```python
from build123d import *

# Parameters (mm, degrees)
SKETCH1_W           = 76.2
SKETCH1_H           = 101.6
SKETCH1_R           = 2.25
BOSS_EXTRUDE1_DEPTH = 3.175


with BuildPart() as part:
    # Sketch1 → Boss-Extrude1 (new body)
    with BuildSketch(Plane(origin=(0, 0, 0), x_dir=(1, 0, 0), z_dir=(0, 1, 0))):
        Rectangle(SKETCH1_W, SKETCH1_H)
        with Locations((-19.05, -41.275)):
            Circle(SKETCH1_R, mode=Mode.SUBTRACT)
        with Locations((19.05, -41.275)):
            Circle(SKETCH1_R, mode=Mode.SUBTRACT)
        with Locations((28.575, -35.56)):
            Circle(SKETCH1_R, mode=Mode.SUBTRACT)
        with Locations((-28.575, -35.56)):
            Circle(SKETCH1_R, mode=Mode.SUBTRACT)
        with Locations((28.575, 35.56)):
            Circle(SKETCH1_R, mode=Mode.SUBTRACT)
        with Locations((19.05, 41.275)):
            Circle(SKETCH1_R, mode=Mode.SUBTRACT)
        with Locations((-28.575, 35.56)):
            Circle(SKETCH1_R, mode=Mode.SUBTRACT)
        with Locations((-19.05, 41.275)):
            Circle(SKETCH1_R, mode=Mode.SUBTRACT)
        with Locations((0, -41.275)):
            Circle(SKETCH1_R, mode=Mode.SUBTRACT)
        with Locations((0, 41.275)):
            Circle(SKETCH1_R, mode=Mode.SUBTRACT)
        with Locations((28.575, 12.7)):
            Circle(SKETCH1_R, mode=Mode.SUBTRACT)
        with Locations((28.575, -12.7)):
            Circle(SKETCH1_R, mode=Mode.SUBTRACT)
        with Locations((22.23, 0)):
            Circle(SKETCH1_R, mode=Mode.SUBTRACT)
    extrude(amount=BOSS_EXTRUDE1_DEPTH)


solid = part.part
```
Here's how the part is built. I have some questions about the finished solid (model axes, mm). Coordinates: 2 decimals unless noted, no trailing zeros. Loops run counter-clockwise (first coordinate to the right, second up) from the corner with the lowest first, then second, coordinate; pieces in that order, holes last. Notation, with made-up numbers: M 41.5,85 L 95.5,85 A33 ccw 95.5,118 Z; hole C 25.5,82.5 d7. An arc over 180 degrees is marked long. One line per item, written item: value.
1. Will these pins go through, and if not, where does the flat tip stop? pin 1 Ø2.5 at (x, z) = (28.575, -12.7) entering from -Y; pin 2 Ø7 at (x, z) = (28.575, -35.56) entering from +Y (3 decimals).
Geometry says:
pin 1: passes through
pin 2: stops at y = 3.175
2. Imagine slicing it at A-A (z = 0). List the corners of the cut face in (x, y) for me (3 decimals), and give its area (3 significant figures).
Geometry says:
outline: M -38.1,0 L 19.98,0 L 19.98,3.175 L -38.1,3.175 Z; M 24.48,0 L 38.1,0 L 38.1,3.175 L 24.48,3.175 Z
area: 228 mm2
3. Please list where these lines run through material, in increasing order: probe 1 along X at (y, z) = (1.5, -35.56) (3 decimals); probe 2 along Z at (x, y) = (-19.05, 2) (3 decimals); probe 3 along X at (y, z) = (0.65, -35).
Geometry says:
probe 1: x = -38.1 to -30.825, -26.325 to 26.325, 30.825 to 38.1
probe 2: z = -50.8 to -43.525, -39.025 to 39.025, 43.525 to 50.8
probe 3: x = -38.1 to -30.75, -26.4 to 26.4, 30.75 to 38.1
4. Imagine slicing it at C-C (y = 2.6). State how many separate pieces and enclosed holes the cut face has, and give its area (3 significant figures).
Geometry says:
separate pieces: 1
enclosed holes: 13
area: 7,540 mm2
5. Imagine slicing it at B-B (z = -35.56). List the corners of the cut face in (x, y) for me (3 decimals).
Geometry says:
outline: M -38.1,0 L -30.825,0 L -30.825,3.175 L -38.1,3.175 Z; M -26.325,0 L 26.325,0 L 26.325,3.175 L -26.325,3.175 Z; M 30.825,0 L 38.1,0 L 38.1,3.175 L 30.825,3.175 Z
6. Thinking about a two-plate mould opening in X: for faces 1 (the flat face through (38.1, 2, 1)), 2 (the cylindrical face through (29.78, 1.57, 10.8)), 3 (the flat face through (-1, 2, 50.8)), 4 (the flat face through (-38.1, 2, 1)), which applies, +X half, -X half, draft (parallel to the pull), parting line (faces both ways), or undercut?
Geometry says:
face 1: +X half
face 2: undercut
face 3: draft
face 4: -X half
